from build123d import *
from OCP.BRepAlgoAPI import BRepAlgoAPI_Cut
from OCP.TopTools import TopTools_ListOfShape

# Parameters (mm, degrees)
BOSS_EXTRUDE1_DEPTH      = 101.413073
BOSS_EXTRUDE1_DEPTH_BACK = 101.413073
CUT_EXTRUDE7_DEPTH       = 115.133874793


with BuildPart() as part:
    # Sketch3 → Boss-Extrude1 (new, two sides: drawn at the far end of the back side and taken through both)
    with BuildSketch(Plane(origin=(0, 0, 0), x_dir=(0, 0, -1), z_dir=(1, 0, 0)).offset(-BOSS_EXTRUDE1_DEPTH_BACK)):
        with BuildLine():
            Line((0, 4.826), (1.984228399, 4.826))
            ThreePointArc((1.984228399, 4.826), (3.199248297, 5.067682484), (4.229292429, 5.75593597))
            Line((4.229292429, 5.75593597), (7.586577723, 9.113221264))
            ThreePointArc((7.586577723, 9.113221264), (7.746562132, 9.955883421), (7.021168939, 10.413572441))
            Line((7.021168939, 10.413572441), (4.090593416, 10.311234489))
            ThreePointArc((4.090593416, 10.311234489), (3.534670322, 10.524633371), (3.302, 11.072770299))
            Line((3.302, 11.072770299), (3.302, 11.70815736))
            ThreePointArc((3.302, 11.70815736), (3.515863072, 12.237487038), (4.037406584, 12.46969317))
            Line((4.037406584, 12.46969317), (10.597084223, 12.698762161))
            ThreePointArc((10.597084223, 12.698762161), (12.104840979, 12.104840979), (12.698762161, 10.597084223))
            Line((12.698762161, 10.597084223), (12.46969317, 4.037406584))
            ThreePointArc((12.46969317, 4.037406584), (12.237487038, 3.515863072), (11.70815736, 3.302))
            Line((11.70815736, 3.302), (11.072770299, 3.302))
            ThreePointArc((11.072770299, 3.302), (10.524633371, 3.534670322), (10.311234489, 4.090593416))
            Line((10.311234489, 4.090593416), (10.413572441, 7.021168939))
            ThreePointArc((10.413572441, 7.021168939), (9.955883421, 7.746562132), (9.113221264, 7.586577723))
            Line((9.113221264, 7.586577723), (5.75593597, 4.229292429))
            ThreePointArc((5.75593597, 4.229292429), (5.067682484, 3.199248297), (4.826, 1.984228399))
            Line((4.826, 1.984228399), (4.826, 0))
            Line((4.826, 0), (2.54, 0))
            ThreePointArc((2.54, 0), (1.796051224, 1.796051224), (0, 2.54))
            Line((0, 2.54), (0, 4.826))
        make_face()
    extrude(amount=BOSS_EXTRUDE1_DEPTH + BOSS_EXTRUDE1_DEPTH_BACK)

    # Mirror1: part across plane


with BuildPart() as part_1:
    add(part.part)
    add(part.part.mirror(Plane.ZX))

    # Mirror2: part across plane


with BuildPart() as part_2:
    add(part_1.part)
    add(part_1.part.mirror(Plane.XY))


with BuildPart() as cut_extrude7_tool:
    # Sketch10 → Cut-Extrude7 (new, through all)
    with BuildSketch(Plane.XY.offset(38.1)):
        Polygon((-76.013073399, -12.7), (-101.413073399, 12.7), (-101.413073399, -12.7), align=None)
        Polygon((-76.013073399, -12.7), (-101.413073399, -12.7), (-101.413073399, 12.7), (-106.454619086, 17.741545687), (-105.960543128, -16.167906454), (-72.545166945, -16.167906454), align=None)
    extrude(amount=-CUT_EXTRUDE7_DEPTH)


with BuildPart() as part_3:
    add(part_2.part)

    # Cut-Extrude7: cut by cut_extrude7_tool, with a tolerance
    cut_extrude7_stock = TopTools_ListOfShape()
    cut_extrude7_stock.Append(part_3.part.wrapped)
    cut_extrude7_tools = TopTools_ListOfShape()
    cut_extrude7_tools.Append(cut_extrude7_tool.part.wrapped)
    cut_extrude7_cut = BRepAlgoAPI_Cut()
    cut_extrude7_cut.SetArguments(cut_extrude7_stock)
    cut_extrude7_cut.SetTools(cut_extrude7_tools)
    cut_extrude7_cut.SetFuzzyValue(0.00001)
    cut_extrude7_cut.Build()
    add(Compound.cast(cut_extrude7_cut.Shape()).solids(), mode=Mode.REPLACE)


solid = part_3.part
The listing builds one solid part. Answer for the finished solid, in the listing's coordinates (mm). A direction names the side the tool comes from. Coordinates: 2 decimals unless noted, no trailing zeros. Put each result on its own line as item: value. Start each with the question number.
1. Consider line 1 (Y direction, x = 0.5, z = -7.25); line 2 (Z direction, x = -48, y = 6.25). Determine where each line is inside the solid, lowest interval first. Write a range as from..to.
2. Which of the six approach directions +Z, -Z, +X, -X, +Y, -Y give full straight-line access (tool end or side, diameter ignored) to faces 1 (the flat face through (7, -4.826, 0)), 2 (the flat face through (4, 0, -4.826)), 3 (the flat face through (0.399, 7.411, 5.884)), 4 (the flat face through (3, 4.826, 0))?
3. For a pull along Y with two mould halves and no side action, classify faces 5 (the flat face through (-88.535, -0.178, 3)), 6 (the flat face through (1.173, 5.931, 7.458)), 7 (the flat face through (7.937, -7.411, 5.884)), 8 (the flat face through (101.413, 0, 3)) as pulls with the +Y half, pulls with the -Y half, needs draft (parallel to the pull), parting line crosses it, or undercut.
4. Flat-ended cylindrical pins translate along their axes: P1, Ø3, axis at x = -14.5, z = 0.5, coming from the -Y side; P2, Ø3, axis at x = 22.5, y = -0.5, coming from the +Z side; P3, Ø2, axis at x = 15, z = -1.5, coming from the +Y side; P4, Ø3, axis at y = 1.5, z = -8.5, coming from the +X side. Find the tip coordinate at first contact, or state that the pin passes through.
Resolved:
1. line 1: y = -12.58..-10.39, -8.78..-5.72, 5.72..8.78, 10.39..12.58
1. line 2: z = -12.55..-10.39, -7.78..-4.72, 4.72..7.78, 10.39..12.55
2. face 1: +X, -X, -Y
2. face 2: -Z, +X, -X
2. face 3: +X, -X
2. face 4: +X, -X, +Y
3. face 5: pulls with the -Y half
3. face 6: undercut
3. face 7: undercut
3. face 8: needs draft
4. P1: stops at y = -4.83
4. P2: stops at z = 4.83
4. P3: stops at y = 4.87
4. P4: passes through
